Source: CAD feature listing. Evaluate the final solid. Frame: model axes, mm. Give positions to 0.01 mm unless a question says otherwise; leave off trailing zeros. Loops run counter-clockwise (first coordinate to the right, second up) from the corner with the lowest first, then second, coordinate; pieces in that order, holes last. Notation, with made-up numbers: (15.5, 25) -> (30.5, 25) arc R28 cw to (30.5, 54) -> close; hole circle Ø6 at (86.25, 3). An arc over 180 degrees is marked (long way). Return JSON: item names as keys, results as strings. Group by question number.
(1) Cut plane A-A on y = 65. Return loops of the section in (x, z), then the cut area to 3 significant figures.
(2) Cut plane B-B on z = 1.8. Return loops of the section in (x, y), then the cut area to 3 significant figures.
(3) Pin query (flat end, axial travel): pin 1 (1.5 mm diameter, centred on x = 128, z = 1, fed in from -Y); pin 2 (1.5 mm diameter, centred on y = 34.5, z = 1.5, fed in from +X); pin 3 (1.5 mm diameter, centred on x = 134, z = 2.5, fed in from -Y). Return the tip coordinate at first contact, or that it passes through.
(4) Ray query, line 1 (X direction, y = 53.5, z = 1.4); line 2 (X direction, y = 69.5, z = 1.8); line 3 (Y direction, x = 148.5, z = 1.95). Return the intervals inside material, ascending. Write a range as from..to.
(5) Cut plane C-C on y = 50.5. Return loops of the section in (x, z).
(6) Cut plane D-D on x = 162. Return loops of the section in (y, z).
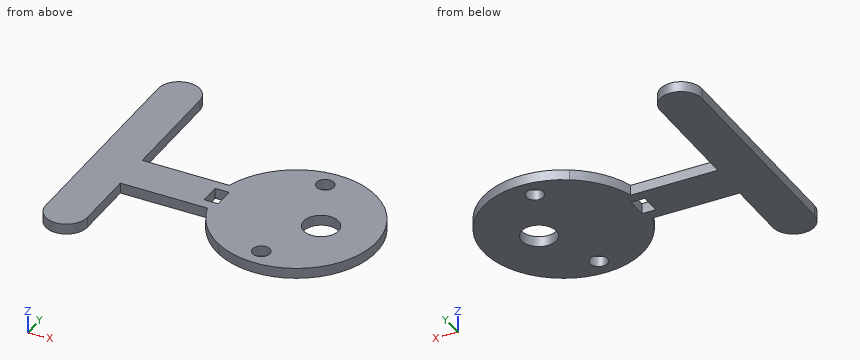
```python
from build123d import *

# Parameters (mm, degrees)
SKETCH_1_R          = 5
SKETCH_1_R_2        = 2.5
EXTRUDE_1_DEPTH     = 3
SKETCH_2_W          = 4
SKETCH_2_H          = 6
CUT_EXTRUDE_1_DEPTH = 3


with BuildPart() as part:
    # 草图1 → 凸台-拉伸1 (new body)
    with BuildSketch(Plane.XY):
        with BuildLine():
            Line((104.204193709, 89.499436202), (104.204193709, 57.999436202))
            Line((104.204193709, 57.999436202), (129.204193709, 57.999436202))
            ThreePointArc((129.204193709, 57.999436202), (133.19157799, 65.772898709), (139.689971603, 71.61214808))
            ThreePointArc((139.689971603, 71.61214808), (174.704134434, 51.947219111), (139.601041877, 32.44147834))
            ThreePointArc((139.601041877, 32.44147834), (133.162334619, 38.267746144), (129.209700495, 45.999436202))
            Line((129.209700495, 45.999436202), (104.204193709, 45.999436202))
            Line((104.204193709, 45.999436202), (104.204193709, 27.999436202))
            ThreePointArc((104.204193709, 27.999436202), (98.204193709, 21.999436202), (92.204193709, 27.999436202))
            Line((92.204193709, 27.999436202), (92.204193709, 89.499436202))
            ThreePointArc((92.204193709, 89.499436202), (98.204193709, 95.499436202), (104.204193709, 89.499436202))
        make_face()
        with Locations((158.704193709, 52.048919583)):
            Circle(SKETCH_1_R, mode=Mode.SUBTRACT)
        with Locations((150.704193709, 69.548919583)):
            Circle(SKETCH_1_R_2, mode=Mode.SUBTRACT)
        with Locations((150.704193709, 34.548919583)):
            Circle(SKETCH_1_R_2, mode=Mode.SUBTRACT)
    extrude(amount=EXTRUDE_1_DEPTH)

    # 草图2 → 切除-拉伸1 (cut)
    with BuildSketch(Plane.XY.offset(3)):
        with Locations((128.704193709, 52.048919583)):
            Rectangle(SKETCH_2_W, SKETCH_2_H)
    extrude(amount=-CUT_EXTRUDE_1_DEPTH, mode=Mode.SUBTRACT)


solid = part.part
```
Answers:
{
 "1": {"outline": "(92.2, 0) -> (104.2, 0) -> (104.2, 3) -> (92.2, 3) -> close; (132.62, 0) -> (170.68, 0) -> (170.68, 3) -> (132.62, 3) -> close", "area": "150 mm²"},
 "2": {"outline": "(92.2, 28) arc R6 ccw to (104.2, 28) -> (104.2, 46) -> (129.21, 46) arc R24.07 ccw to (139.6, 32.44) arc R23 ccw (long way) to (139.69, 71.61) arc R24.08 ccw to (129.2, 58) -> (104.2, 58) -> (104.2, 89.5) arc R6 ccw to (92.2, 89.5) -> close; hole (126.7, 49.05) -> (130.7, 49.05) -> (130.7, 55.05) -> (126.7, 55.05) -> close; hole circle Ø5 at (150.7, 34.55); hole circle Ø5 at (150.7, 69.55); hole circle Ø10 at (158.7, 52.05)", "area": "2,670 mm²"},
 "3": {"pin 1": "y = 46", "pin 2": "x = 167.47", "pin 3": "y = 36.4"},
 "4": {"line 1": "92.2..126.7, 130.7..153.92, 163.49..174.66", "line 2": "92.2..104.2, 136.76..148.2, 153.2..166.63", "line 3": "29.22..33.37, 35.73..68.37, 70.73..74.78"},
 "5": {"outline": "(92.2, 0) -> (126.7, 0) -> (126.7, 3) -> (92.2, 3) -> close; (130.7, 0) -> (153.95, 0) -> (153.95, 3) -> (130.7, 3) -> close; (163.46, 0) -> (174.66, 0) -> (174.66, 3) -> (163.46, 3) -> close"},
 "6": {"outline": "(31.43, 0) -> (48.29, 0) -> (48.29, 3) -> (31.43, 3) -> close; (55.81, 0) -> (72.57, 0) -> (72.57, 3) -> (55.81, 3) -> close"}
}
